Check sheet for the drawn part. Datum: minimum x, y, z corner. Units: mm. A direction names the side the tool comes from. Round coordinates to 2 decimals unless told otherwise and drop trailing zeros. Write each loop counter-clockwise with the first axis right and the second up, starting at its lowest first coordinate (ties: lowest second). Pieces come first, ordered by that corner, then holes. Notation, with made-up numbers: M 10,72.5 L 67,72.5 A30 cw 67,111.5 Z; hole C 62,73 d4. An arc over 180 degrees is marked long. Answer in a Markdown table with one row per item. Add a question column.
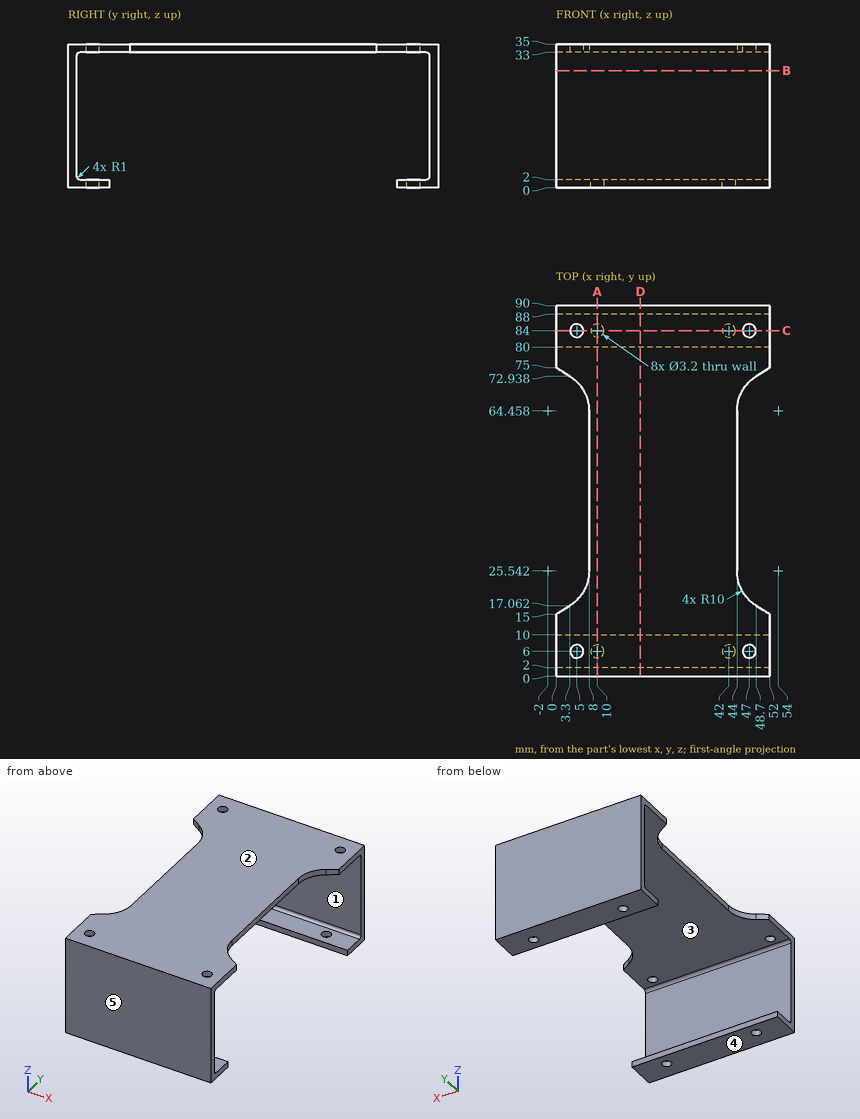
Item 1: Section check C-C, the plane y = 84. Record the boundary of the cut face in (x, z).
Item 2: Mould release check, pull along Z, two halves, no side actions. Record for the marked faces 3, 4 and 5: +Z half, -Z half, draft (parallel to the pull), parting line (faces both ways), or undercut.
Item 3: Section check A-A, the plane x = 10. Record the boundary of the cut face in (y, z), and give its area (3 significant figures).
Item 4: Access from +Z, -Z, +X, -X, +Y, -Y to the whole of each face (thin tool, end or side, straight path). Record for the marked faces 1 and 2.
Item 5: Section check B-B, the plane z = 28.5. Record the boundary of the cut face in (x, y).
Item 6: Gauge pin test, flat ends, axial feed: pin 1 Ø3 at (x, y) = (10, 6) entering from -Z; pin 2 Ø2 at (y, z) = (36.5, 34) entering from +X. Record the tip position at first contact, or that the pin passes through.
Item 7: Section check D-D, the plane x = 20.5. Record the boundary of the cut face in (y, z).
Item 8: Scan lines: probe 1 along X at (y, z) = (84, 1.25); probe 2 along Y at (x, z) = (22.5, 32); probe 3 along Z at (x, y) = (3, 7.5). Record each from-to range of solid material in increasing order. Write a range as from..to.
Result sheet:
| question | item | result |
|---|---|---|
| 1 | outline | M 0,0 L 8.4,0 L 8.4,2 L 0,2 Z; M 0,33 L 3.4,33 L 3.4,35 L 0,35 Z; M 6.6,33 L 45.4,33 L 45.4,35 L 6.6,35 Z; M 11.6,0 L 40.4,0 L 40.4,2 L 11.6,2 Z; M 43.6,0 L 52,0 L 52,2 L 43.6,2 Z; M 48.6,33 L 52,33 L 52,35 L 48.6,35 Z |
| 2 | face 3 | undercut |
| 2 | face 4 | -Z half |
| 2 | face 5 | draft |
| 3 | outline | M 0,0 L 4.4,0 L 4.4,2 L 3,2 A1 cw 2,3 L 2,32 A1 cw 3,33 L 87,33 A1 cw 88,32 L 88,3 A1 cw 87,2 L 85.6,2 L 85.6,0 L 90,0 L 90,35 L 0,35 Z; M 7.6,0 L 10,0 L 10,2 L 7.6,2 Z; M 80,0 L 82.4,0 L 82.4,2 L 80,2 Z |
| 3 | area | 332 mm^2 |
| 4 | face 1 | +X, -X |
| 4 | face 2 | +Z, +X, -X, +Y, -Y |
| 5 | outline | M 0,0 L 52,0 L 52,2 L 0,2 Z; M 0,88 L 52,88 L 52,90 L 0,90 Z |
| 6 | pin 1 | stops at z = 33 |
| 6 | pin 2 | stops at x = 44 |
| 7 | outline | M 0,0 L 10,0 L 10,2 L 3,2 A1 cw 2,3 L 2,32 A1 cw 3,33 L 87,33 A1 cw 88,32 L 88,3 A1 cw 87,2 L 80,2 L 80,0 L 90,0 L 90,35 L 0,35 Z |
| 8 | probe 1 | x = 0..8.4, 11.6..40.4, 43.6..52 |
| 8 | probe 2 | y = 0..2, 88..90 |
| 8 | probe 3 | z = 0..2, 33..35 |
